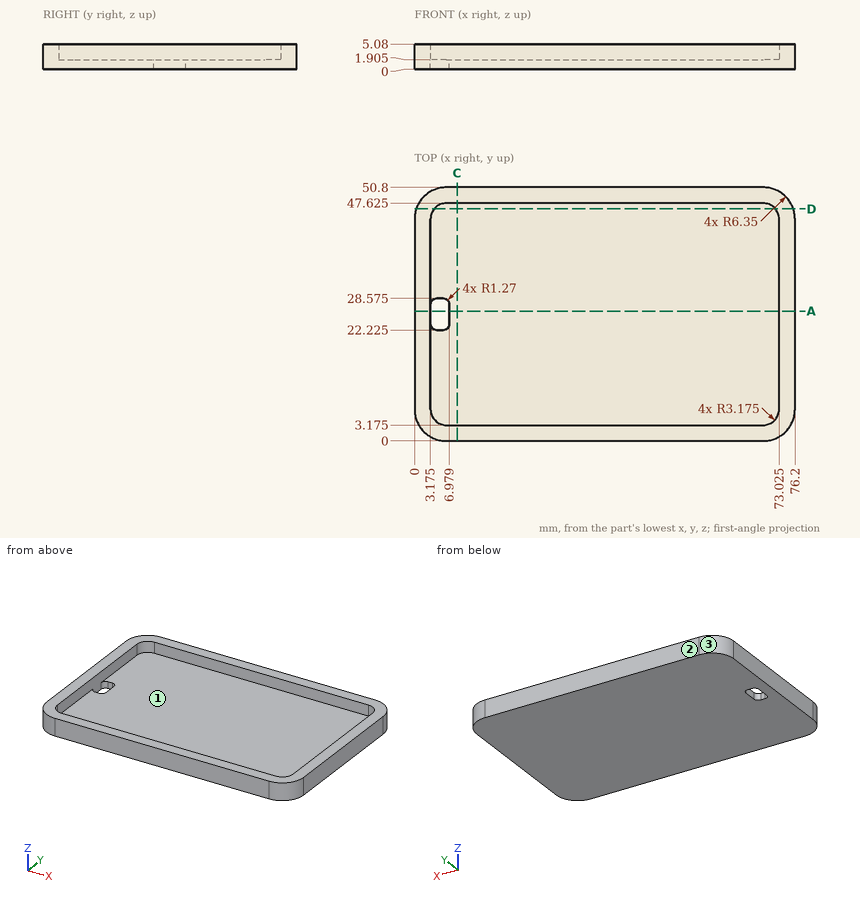
Can you work these out from the drawing? Everything is in mm from the part's minimum corner. Round coordinates to 2 decimals unless told otherwise and drop trailing zeros. Write each loop counter-clockwise with the first axis right and the second up, starting at its lowest first coordinate (ties: lowest second). Pieces come first, ordered by that corner, then holes. Notation, with made-up numbers: (-35, 78.5) - (15, 78.5) arc R11 cw to (15, 84.5) - close; hole circle Ø8 at (9.5, -29.5). An arc over 180 degrees is marked (long way). Put each result on its own line as item: value. Start each with the question number.
(1) I want a section at A-A, the plane y = 26. Please give me the cut outline in (x, z) (1 decimal).
(2) I need wall thicknesses on probe 1 along X at (y, z) = (22, 4.8) (1 decimal); probe 2 along Y at (x, z) = (26, 2.7) (1 decimal); probe 3 along Z at (x, y) = (33.5, 11.5) (1 decimal). Which ranges of each line are inside material? Lowest first, please.
(3) I want a section at D-D, the plane y = 46.5. Please give me the cut outline in (x, z) (1 decimal), plus the area to 3 significant figures.
(4) Thinking about a two-plate mould opening in X: for the marked faces 1, 2 and 3, which applies, released by +X, released by -X, zero draft, split by the parting line, or undercut?
(5) I want a section at C-C, the plane x = 8.5. Please give me the cut outline in (y, z) (1 decimal).
(6) Will these pins go through, and if not, where does the flat tip stop? pin 1 (22 mm diameter, centred on x = 33, y = 22, fed in from +Z) (3 decimals); pin 2 (1 mm diameter, centred on x = 5.5, z = 1, fed in from +Y); pin 3 (0.6 mm diameter, centred on x = 5, z = 1, fed in from -Y).
Here are the results:
1. outline: (0, 0) - (3.2, 0) - (3.2, 5.1) - (0, 5.1) - close; (7, 0) - (76.2, 0) - (76.2, 5.1) - (73, 5.1) - (73, 1.9) - (7, 1.9) - close
2. probe 1: x = 0 to 3.2, 73 to 76.2
2. probe 2: y = 0 to 3.2, 47.6 to 50.8
2. probe 3: z = 0 to 1.9
3. outline: (0.3, 0) - (75.9, 0) - (75.9, 5.1) - (72.3, 5.1) - (72.3, 1.9) - (3.9, 1.9) - (3.9, 5.1) - (0.3, 5.1) - close
3. area: 167 mm^2
4. face 1: undercut
4. face 2: zero draft
4. face 3: released by -X
5. outline: (0, 0) - (50.8, 0) - (50.8, 5.1) - (47.6, 5.1) - (47.6, 1.9) - (3.2, 1.9) - (3.2, 5.1) - (0, 5.1) - close
6. pin 1: stops at z = 1.905
6. pin 2: stops at y = 50.79
6. pin 3: stops at y = 0.09
